```python
from build123d import *

# Parameters (mm, degrees)
F1_DEPTH = 3.175


with BuildPart() as f1:
    # F0 (on Front) → F1 (new body)
    with BuildSketch(Plane.XZ):
        with BuildLine():
            Line((0, 101.6), (0, 0))
            Line((0, 0), (95.25, 0))
            Line((95.25, 0), (95.25, 101.6))
            Line((95.25, 101.6), (65.585512, 101.6))
            ThreePointArc((65.585512, 101.6), (61.919338, 100.434753), (59.598675, 97.366667))
            ThreePointArc((59.598675, 97.366667), (47.625, 88.9), (35.651325, 97.366667))
            ThreePointArc((35.651325, 97.366667), (33.330662, 100.434753), (29.664488, 101.6))
            Line((29.664488, 101.6), (0, 101.6))
        make_face()
    extrude(amount=F1_DEPTH)


solid = f1.part
```
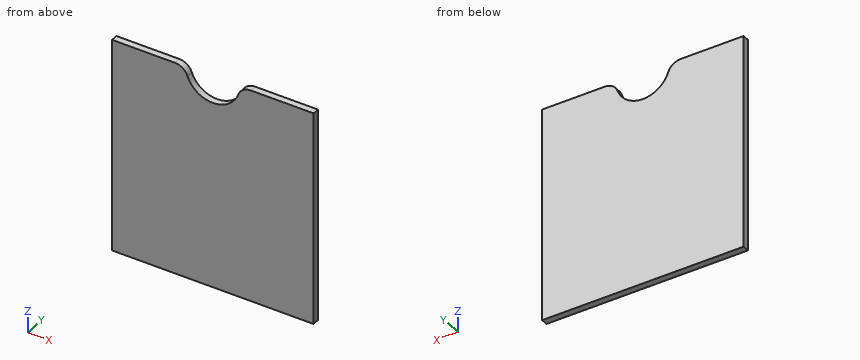
Input: part model. Units: mm. Frame: model coordinates. Round coordinates to 2 decimals unless told otherwise and drop trailing zeros. Loops run counter-clockwise (first coordinate to the right, second up) from the corner with the lowest first, then second, coordinate; pieces in that order, holes last. Notation, with made-up numbers: (20, -3.5) -> (56, -3.5) arc R31 ccw to (56, 33.5) -> close; hole circle Ø1 at (15.25, 67). An arc over 180 degrees is marked (long way). Use one line per item in the form item = value. Start each with the question number.
Item 1: Section query B-B on z = 94. Return the cut outline in (x, y) (3 decimals), then the cut area to 3 significant figures.
Item 2: Material intervals for L1, parallel to Z at x = 37, y = -0.85; L2, parallel to Z at x = 53, y = -1.8, sorted ascending. Write a range as from..to.
Item 3: Section query A-A on y = -0.9. Return the cut outline in (x, z) (3 decimals), then the cut area to 3 significant figures.
Item 4: Contact query for a flat-ended pin moving along its axis: pin 1 Ø12 at (x, z) = (15, 11) entering from +Y. Output: stop coordinate, or through.
Item 5: Section query C-C on x = 56. Return the cut outline in (y, z) (3 decimals), then the cut area to 3 significant figures.
Ans:
q1.outline = (0, -3.175) -> (37.45, -3.175) -> (37.45, 0) -> (0, 0) -> close; (57.8, -3.175) -> (95.25, -3.175) -> (95.25, 0) -> (57.8, 0) -> close
q1.area = 238 mm^2
q2.L1 = 0..94.64
q2.L2 = 0..90.09
q3.outline = (0, 0) -> (95.25, 0) -> (95.25, 101.6) -> (65.586, 101.6) arc R6.35 ccw to (59.599, 97.367) arc R12.7 cw to (35.651, 97.367) arc R6.35 ccw to (29.664, 101.6) -> (0, 101.6) -> close
q3.area = 9,410 mm^2
q4.pin_1 = 0
q5.outline = (-3.175, 0) -> (0, 0) -> (0, 92.053) -> (-3.175, 92.053) -> close
q5.area = 292 mm^2
